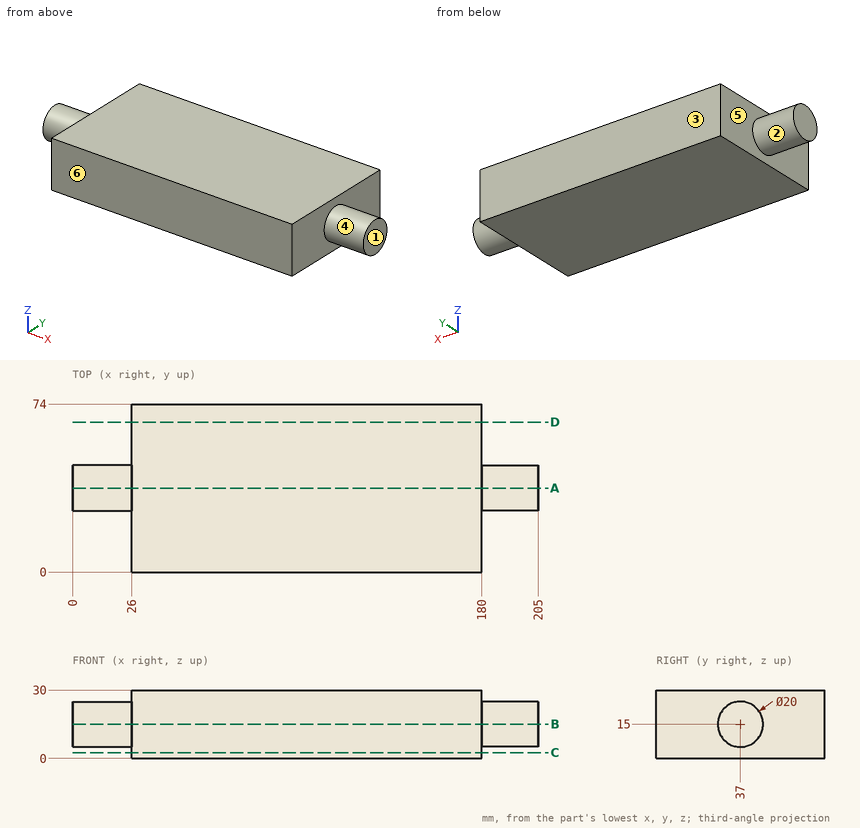
Answer from the drawing. Dimensions are ordinates in mm from the lowest x, y and z of the part. A direction names the side the tool comes from. Coordinates: 2 decimals unless noted, no trailing zeros. Loops run counter-clockwise (first coordinate to the right, second up) from the corner with the lowest first, then second, coordinate; pieces in that order, holes last. Notation, with made-up numbers: (47, -7.5) - (86, -7.5) arc R19 ccw to (86, -0.5) - close; hole circle Ø6 at (-32.75, 75.25). An arc over 180 degrees is marked (long way). Answer in a Markdown table with one row per item.
1. Find section D-D, the plane y = 66. Write down the section's boundary in (x, z).
Conclusion:
| item | result |
|---|---|
| outline | (26, 0) - (180, 0) - (180, 30) - (26, 30) - close |
2. Find section C-C, the plane z = 2.5. Write down the section's boundary in (x, y), then the cut area to 3 significant figures.
Conclusion:
| item | result |
|---|---|
| outline | (26, 0) - (180, 0) - (180, 74) - (26, 74) - close |
| area | 11,400 mm² |
3. Which of the six approach directions +Z, -Z, +X, -X, +Y, -Y give full straight-line access (tool end or side, diameter ignored) to the marked faces 1 and 2?
Conclusion:
| item | result |
|---|---|
| face 1 | +Z, -Z, +X, +Y, -Y |
| face 2 | -X |
4. Find section A-A, the plane y = 37. Write down the section's boundary in (x, z).
Conclusion:
| item | result |
|---|---|
| outline | (0, 5) - (26, 5) - (26, 0) - (180, 0) - (180, 5) - (205, 5) - (205, 25) - (180, 25) - (180, 30) - (26, 30) - (26, 25) - (0, 25) - close |
5. Straight lines are drawn through the part: line 1 (X direction, y = 17, z = 4.25); line 2 (Y direction, x = 186.5, z = 18.25); line 3 (Y direction, x = 188.5, z = 18.5). For each, find the intervals that lie inside material, in ascending order.
Conclusion:
| item | result |
|---|---|
| line 1 | x = 26 to 180 |
| line 2 | y = 27.54 to 46.46 |
| line 3 | y = 27.63 to 46.37 |
6. Given pin 1 (2 mm diameter, centred on y = 50, z = 25.5, fed in from +X), flat-ended and moving along its own axis, determine where the tip first touches the part or whether it passes through.
Conclusion:
| item | result |
|---|---|
| pin 1 | stops at x = 180 |
7. Determine the mould class of the marked faces 3, 4, 5 and 6 for opening direction Y: +Y half, -Y half, draft (parallel to the pull), parting line (faces both ways), or undercut.
Conclusion:
| item | result |
|---|---|
| face 3 | +Y half |
| face 4 | parting line |
| face 5 | draft |
| face 6 | -Y half |
8. Find section B-B, the plane z = 15. Write down the section's boundary in (x, y).
Conclusion:
| item | result |
|---|---|
| outline | (0, 27) - (26, 27) - (26, 0) - (180, 0) - (180, 27) - (205, 27) - (205, 47) - (180, 47) - (180, 74) - (26, 74) - (26, 47) - (0, 47) - close |
